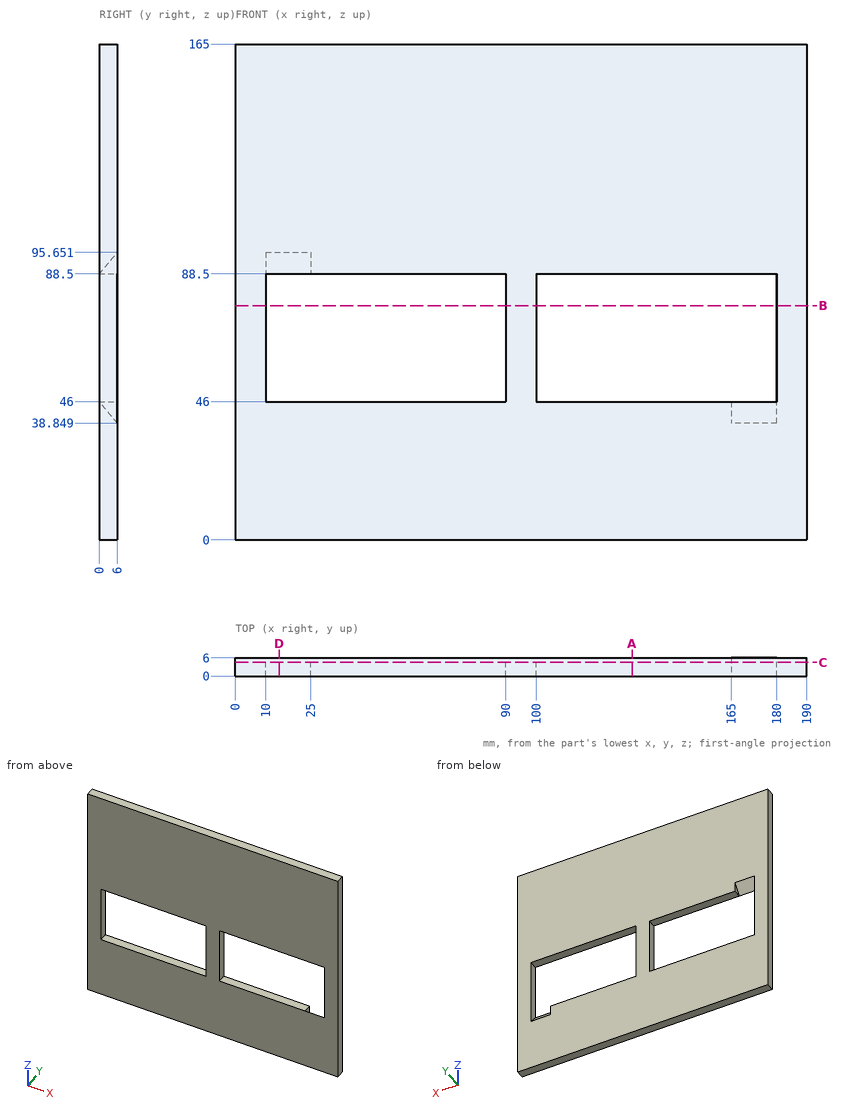
The figure shows three views and two pictorial views of one solid part (mm, origin at its lowest corner). Answer the questions. Coordinates: 2 decimals unless noted, no trailing zeros. Write each loop counter-clockwise with the first axis right and the second up, starting at its lowest first coordinate (ties: lowest second). Pieces come first, ordered by that corner, then holes. Notation, with made-up numbers: (9, 80.25) -> (67, 80.25) arc R13 cw to (67, 100.25) -> close; hole circle Ø3 at (45, 18). An arc over 180 degrees is marked (long way). Answer as a JSON object with one key per item and string values.
Q1. Consider line 1 (X direction, y = 0.75, z = 76); line 2 (Z direction, x = 149.5, y = 5.25); line 3 (Z direction, x = 21, y = 5.5) (1 decimal). Determine where each line is inside the solid, lowest interval first. Write a range as [from, to].
The answers:
{"line 1": "x = [0, 10], [90, 100], [180, 190]", "line 2": "z = [0, 46], [88.5, 165]", "line 3": "z = [0, 46], [95.1, 165]"}
Q2. The part is cut by section A-A on x = 132. Give the vertices of the cut face in (y, z).
The answers:
{"outline": "(0, 0) -> (6, 0) -> (6, 46) -> (0, 46) -> close; (0, 88.5) -> (6, 88.5) -> (6, 165) -> (0, 165) -> close"}
Q3. The part is cut by section B-B on z = 78. Give the vertices of the cut face in (x, y), then the cut area to 3 significant figures.
The answers:
{"outline": "(0, 0) -> (10, 0) -> (10, 6) -> (0, 6) -> close; (90, 0) -> (100, 0) -> (100, 6) -> (90, 6) -> close; (180, 0) -> (190, 0) -> (190, 6) -> (180, 6) -> close", "area": "180 mm2"}
Q4. The part is cut by section C-C on y = 4.5. Give the vertices of the cut face in (x, z), then the cut area to 3 significant figures.
The answers:
{"outline": "(0, 0) -> (190, 0) -> (190, 165) -> (0, 165) -> close; hole (10, 46) -> (90, 46) -> (90, 88.5) -> (25, 88.5) -> (25, 93.86) -> (10, 93.86) -> close; hole (100, 46) -> (165, 46) -> (165, 40.64) -> (180, 40.64) -> (180, 88.5) -> (100, 88.5) -> close", "area": "24,400 mm2"}
Q5. The part is cut by section D-D on x = 14.5. Give the vertices of the cut face in (y, z).
The answers:
{"outline": "(0, 0) -> (6, 0) -> (6, 46) -> (0, 46) -> close; (0, 88.5) -> (6, 95.65) -> (6, 165) -> (0, 165) -> close"}
